Source: CAD feature listing. Evaluate the final solid. Frame: model axes, mm. Face numbers are marked on the shaded views. A direction names the side the tool comes from. Coordinates: 2 decimals unless noted, no trailing zeros. Loops run counter-clockwise (first coordinate to the right, second up) from the corner with the lowest first, then second, coordinate; pieces in that order, holes last. Notation, with made-up numbers: (-35, 49) - (2, 49) arc R13 cw to (2, 71) - close; hole circle Ø1 at (61.5, 11.25). An arc over 180 degrees is marked (long way). Use CSV: the item, a comma, the result in double quotes. Start each with the question number.
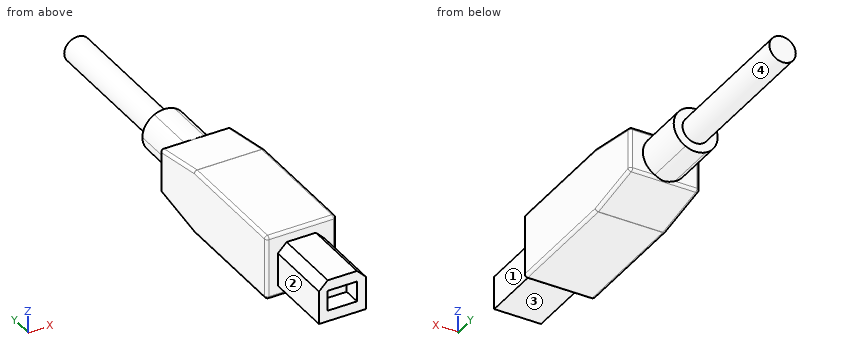
```python
from build123d import *

# Parameters (mm, degrees)
F0_W          = 8
F0_H          = 7.2
F0_W_2        = 5
F0_H_2        = 3.5
F1_DEPTH      = 12
F2_DEPTH      = 9
F3_SIZE       = 1.5
F0_W_3        = 12
F0_H_3        = 11
F4_DEPTH      = 31
F5_SIZE2      = 1.75
F5_SIZE       = 10
F5_2_SIZE2    = 1.75
F5_2_SIZE     = 10
F6_R          = 0.5
F8_DEPTH      = 9
F8_DEPTH_BACK = 0.2288594728
F9_R          = 2.25
F10_DEPTH     = 25.4


with BuildPart() as f1:
    # F0 (on Front) → F1 (new body)
    with BuildSketch(Plane.XZ):
        Rectangle(F0_W, F0_H)
        Rectangle(F0_W_2, F0_H_2, mode=Mode.SUBTRACT)
    extrude(amount=F1_DEPTH)

    # F0 (on Front) → F2 (join)
    with BuildSketch(Plane.XZ):
        Rectangle(F0_W_2, F0_H_2)
    extrude(amount=F2_DEPTH)

    # F3
    f3_edges = [f1.edges().sort_by_distance(p)[0] for p in [
        (-4, -6, 3.6),
        (4, -6, 3.6),
    ]]
    chamfer(f3_edges, length=F3_SIZE)

    # F0 (on Front) → F4 (join)
    with BuildSketch(Plane.XZ):
        Rectangle(F0_W_3, F0_H_3)
        Rectangle(F0_W, F0_H, mode=Mode.SUBTRACT)
        Rectangle(F0_W, F0_H)
        Rectangle(F0_W_2, F0_H_2, mode=Mode.SUBTRACT)
        Rectangle(F0_W_2, F0_H_2)
    extrude(amount=-F4_DEPTH)

    # F5
    f5_edges = [f1.edges().sort_by_distance(p)[0] for p in [
        (0, 31, 5.5),
    ]]
    f5_side = f1.faces().sort_by_distance((0, 15.5, 5.5))[0]
    chamfer(f5_edges, length=F5_SIZE, length2=F5_SIZE2, reference=f5_side)

    # F5#2
    f5_2_edges = [f1.edges().sort_by_distance(p)[0] for p in [
        (0, 31, -5.5),
    ]]
    f5_2_side = f1.faces().sort_by_distance((0, 15.5, -5.5))[0]
    chamfer(f5_2_edges, length=F5_2_SIZE, length2=F5_2_SIZE2, reference=f5_2_side)

    # F6
    f6_edges = [f1.edges().sort_by_distance(p)[0] for p in [
        (-6, 31, 0),
        (-6, 26, -4.625),
        (-6, 26, 4.625),
        (-6, 10.5, -5.5),
        (-6, 10.5, 5.5),
        (-6, 0, 0),
        (6, 31, 0),
        (6, 26, -4.625),
        (6, 26, 4.625),
        (6, 10.5, -5.5),
        (6, 10.5, 5.5),
        (6, 0, 0),
        (0, 21, 5.5),
        (0, 0, 5.5),
        (0, 21, -5.5),
        (0, 0, -5.5),
        (0, 31, -3.75),
        (0, 31, 3.75),
    ]]
    fillet(f6_edges, radius=F6_R)

    # F7 (on face) → F8 (join, two sides)
    with BuildSketch(Plane(origin=(0, 31, 0), x_dir=(-1, 0, 0), z_dir=(0, 1, 0))) as f8_sk:
        with BuildLine():
            Line((-1.7246031672, 3.3299014874), (1.7246031672, 3.3299014874))
            ThreePointArc((1.7246031672, 3.3299014874), (0, 3.75), (-1.7246031672, 3.3299014874))
        make_face()
        with BuildLine():
            ThreePointArc((1.7246031672, -3.3299014874), (3.203885288, -1.9487480754), (3.75, 0))
            ThreePointArc((3.75, 0), (3.203885288, 1.9487480754), (1.7246031672, 3.3299014874))
            Line((1.7246031672, 3.3299014874), (-1.7246031672, 3.3299014874))
            ThreePointArc((-1.7246031672, 3.3299014874), (-3.75, 0), (-1.7246031672, -3.3299014874))
            Line((-1.7246031672, -3.3299014874), (1.7246031672, -3.3299014874))
        make_face()
        with BuildLine():
            ThreePointArc((-1.7246031672, -3.3299014874), (0, -3.75), (1.7246031672, -3.3299014874))
            Line((1.7246031672, -3.3299014874), (-1.7246031672, -3.3299014874))
        make_face()
    extrude(amount=F8_DEPTH)
    extrude(f8_sk.sketch, amount=-F8_DEPTH_BACK)

    # F9 (on face) → F10 (join)
    with BuildSketch(Plane(origin=(0, 40, 0), x_dir=(-1, 0, 0), z_dir=(0, 1, 0))):
        Circle(F9_R)
    extrude(amount=F10_DEPTH)


solid = f1.part
```
(1) Ray query, line 1 (Y direction, x = 0.5, z = 0.5); line 2 (Z direction, x = 1.75, y = -2); line 3 (Y direction, x = -2.5, z = -2.25). Return the intervals inside material, ascending. Write a range as [from, to].
(2) Pin query (flat end, axial travel): pin 1 Ø3 at (y, z) = (-8.5, 0) entering from -X; pin 2 Ø3.5 at (x, y) = (0.5, -10) entering from +Z; pin 3 Ø6.5 at (y, z) = (-4, 0.5) entering from +X. Return the tip coordinate at first contact, or that it passes through.
(3) Section C-C on y = -7. Output: boundary loops of the cut face in (x, z), plus the area to 4 significant figures.
(4) Section D-D on y = 60. Output: boundary loops of the cut face in (x, z), plus the area to 3 significant figures.
(5) Section B-B on x = 0. Output: boundary loops of the cut face in (y, z).
(6) Reachability of the marked faces 1, 2, 3 and 4 from +Z, -Z, +X, -X, +Y, -Y: full face, straight path, thin tool, end or side. Return the list, or none.
(7) Section A-A on y = 39. Output: boundary loops of the cut face in (x, z).
Solution:
1,line 1,"y = [-9, 65.4]"
1,line 2,"z = [-3.6, 3.6]"
1,line 3,"y = [-12, 40]"
2,pin 1,"stops at x = -4"
2,pin 2,"stops at z = 3.6"
2,pin 3,"stops at x = 4"
3,outline,"(-4, -3.6) - (4, -3.6) - (4, 2.1) - (2.5, 3.6) - (-2.5, 3.6) - (-4, 2.1) - close"
3,area,"55.35 mm²"
4,outline,"circle Ø4.5 at (0, 0)"
4,area,"15.9 mm²"
5,outline,"(-12, -3.6) - (0, -3.6) - (0, -5) arc R0.5 ccw to (0.5, -5.5) - (20.96, -5.5) arc R0.5 ccw to (21.04, -5.49) - (30.59, -3.82) arc R0.5 ccw to (30.77, -3.75) - (40, -3.75) - (40, -2.25) - (65.4, -2.25) - (65.4, 2.25) - (40, 2.25) - (40, 3.75) - (30.77, 3.75) arc R0.5 ccw to (30.59, 3.82) - (21.04, 5.49) arc R0.5 ccw to (20.96, 5.5) - (0.5, 5.5) arc R0.5 ccw to (0, 5) - (0, 3.6) - (-12, 3.6) - (-12, 1.75) - (-9, 1.75) - (-9, -1.75) - (-12, -1.75) - close"
6,face 1,"+Z, -Z, +X, -Y"
6,face 2,"+Z, -Z, -X, -Y"
6,face 3,"-Z, +X, -X, -Y"
6,face 4,"+Y"
7,outline,"circle Ø7.5 at (0, 0)"
